Geometry check sheet. Reference: the model listing, model coordinates, mm. Round coordinates to 2 decimals unless told otherwise and drop trailing zeros. Order: outer loops, then holes, each group sorted by start corner. A loop starts at its lowest first (then second) coordinate and runs counter-clockwise, first axis right, second up.
(1) Material ranges on line 1 along Z through (x, y) = (-61.5, 0.1); line 2 along X through (y, z) = (0.1, 3); line 3 along Y through (x, z) = (-1.5, 2.25), recorded low to high.
(2) Go/stop test with a flat-tipped pin: pin 1 (7.5 mm diameter, centred on x = 0.5, z = 0, fed in from +Y). Record where the tip stops, or that it passes through.
(3) Sectioned sample at B-B (x = -49.5). Record the boundary of the cut face in (y, z), plus the area to 3 significant figures.
from build123d import *

# Parameters (mm, degrees)
BOSS_EXTRUDE1_DEPTH = 0.2032
SKETCH2_R           = 4.826
CUT_EXTRUDE1_DEPTH  = 0.00254
FILLET1_R           = 2.54


with BuildPart() as part:
    # Sketch1 → Boss-Extrude1 (new body)
    with BuildSketch(Plane(origin=(0, 0, 0), x_dir=(1, 0, 0), z_dir=(0, 1, 0))):
        Polygon((-120.65, -0.635), (-127, -0.635), (-127, 0.635), (-120.65, 0.635), (-120.65, 3.175), (-127, 3.175), (-127, 4.445), (-120.65, 4.445), (-120.65, 5.588), (-108.748705113, 5.588), (-12.192, 5.588), (-7.62, 6.985), (6.35, 6.985), (6.35, -6.985), (-7.62, -6.985), (-12.192, -5.588), (-108.748705113, -5.588), (-120.65, -5.588), (-120.65, -4.445), (-127, -4.445), (-127, -3.175), (-120.65, -3.175), align=None)
    extrude(amount=BOSS_EXTRUDE1_DEPTH)

    # Sketch2 → Cut-Extrude1 (cut)
    with BuildSketch(Plane(origin=(0, 0.2032, 0), x_dir=(1, 0, 0), z_dir=(0, 1, 0))):
        Circle(SKETCH2_R)
    extrude(amount=-CUT_EXTRUDE1_DEPTH, mode=Mode.SUBTRACT)

    # Fillet1
    fillet1_edges = [part.edges().sort_by_distance(p)[0] for p in [
        (6.35, 0.1016, -6.985),
        (6.35, 0.1016, 6.985),
    ]]
    fillet(fillet1_edges, radius=FILLET1_R)


solid = part.part
Answer below:
1. line 1: z = -5.59 to 5.59
1. line 2: x = -120.65 to 6.35
1. line 3: y = 0 to 0.2
2. pin 1: stops at y = 0.2
3. outline: (0, -5.59) - (0.2, -5.59) - (0.2, 5.59) - (0, 5.59) - close
3. area: 2.27 mm2
